```python
from build123d import *

# Parameters (mm, degrees)
EXTRUDE_1_DEPTH        = 20
SKETCH_6_R             = 5
SKETCH_6_R_2           = 2
CUT_EXTRUDE_2_DEPTH    = 2
CHAMFER_2_SIZE         = 4
CHAMFER_3_SIZE         = 0.5
HOLE_WIZARD_M3_1_D     = 2.5
HOLE_WIZARD_M3_1_DEPTH = 7.5
HOLE_WIZARD_M3_1_TIP   = 0.751075774


with BuildPart() as part:
    # 草图1 → 凸台-拉伸1 (new body)
    with BuildSketch(Plane.XY):
        Polygon((0, 3), (0, 0), (-3, 0), (-3, 15), (6, 15), (6, 3), align=None)
    extrude(amount=EXTRUDE_1_DEPTH)

    # 草图6 → 切除-拉伸2 (cut)
    with BuildSketch(Plane.ZY.offset(3)):
        with Locations(Location((10, 9, 0), (0, 0, 270))):
            Circle(SKETCH_6_R)
        with Locations(Location((10, 9, 0), (0, 0, 270))):
            Circle(SKETCH_6_R_2, mode=Mode.SUBTRACT)
    extrude(amount=-CUT_EXTRUDE_2_DEPTH, mode=Mode.SUBTRACT)

    # 倒角2
    chamfer_2_edges = [part.edges().sort_by_distance(p)[0] for p in [
        (1.5, 15, 20),
        (1.5, 15, 0),
    ]]
    chamfer(chamfer_2_edges, length=CHAMFER_2_SIZE)

    # 倒角3
    chamfer_3_edges = [part.edges().sort_by_distance(p)[0] for p in [
        (6, 3, 10),
        (0, 0, 10),
        (-3, 14, 10),
        (-3, 11, 10),
    ]]
    chamfer(chamfer_3_edges, length=CHAMFER_3_SIZE)

    # M3 螺纹孔1
    with Locations(Plane(origin=(0, 3, 0), x_dir=(-1, 0, 0), z_dir=(0, -1, 0))):
        with Locations((-2.5, -5), (-2.5, -15)):
            Hole(HOLE_WIZARD_M3_1_D / 2, depth=HOLE_WIZARD_M3_1_DEPTH)
            with Locations((0, 0, -(HOLE_WIZARD_M3_1_DEPTH + HOLE_WIZARD_M3_1_TIP / 2))):  # 118° drill point
                Cone(0, HOLE_WIZARD_M3_1_D / 2, HOLE_WIZARD_M3_1_TIP, mode=Mode.SUBTRACT)


solid = part.part
```
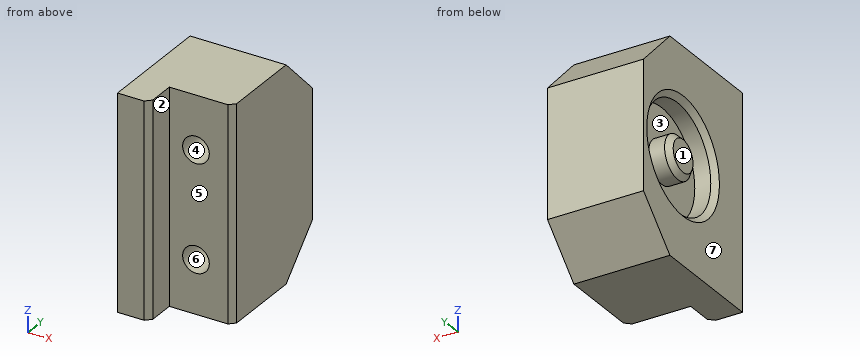
Design review of the part built by this model. Coordinates are the model's own, in mm. Face numbers are marked on the shaded views. A direction names the side the tool comes from. Coordinates: 2 decimals unless noted, no trailing zeros. Loops run counter-clockwise (first coordinate to the right, second up) from the corner with the lowest first, then second, coordinate; pieces in that order, holes last. Notation, with made-up numbers: (-2.5, -31.5) - (8.5, -31.5) arc R20 cw to (8.5, -12.5) - close; hole circle Ø3 at (85, 50.25). An arc over 180 degrees is marked (long way). Use CSV: the item, a comma, the result in double quotes. Start each with the question number.
1) Consider section D-D on y = 3.25. Write out the cut boundary in (x, z), then the cut area to 3 significant figures.
2) Tool access review of the marked faces 1, 2 and 3: name each direction out of +Z, -Z, +X, -X, +Y, -Y from which nothing blocks a thin tool from reaching the whole face with its end or side.
3) Consider section C-C on z = 1.75. Write out the cut boundary in (x, y).
4) Wall thickness on L1, parallel to Z at x = 2.5, y = 6; L2, parallel to X at y = 6.5, z = 15; L3, parallel to Z at x = -1.85, y = 9: over which ranges is each line inside the solid? List them lowest first. Write a range as from..to.
5) Consider section A-A on y = 9. Write out the cut boundary in (x, z), then the cut area to 3 significant figures.
6) Consider section B-B on x = 5. Write out the cut boundary in (y, z).
7) For pin 1 Ø3 at (x, z) = (5, 3) entering from -Y; pin 2 Ø1 at (y, z) = (10.5, 14) entering from -X; pin 3 Ø1.5 at (x, z) = (2.5, 5) entering from -Y, all flat-tipped, find the tip position at first contact; note any pin that passes through.
8) The part is to be moulded in two halves that separate along X. For the marked faces 4, 5, 6 and 7, say which applies: +X half, -X half, draft (parallel to the pull), parting line (faces both ways), or undercut.
Geometry says:
1,outline,"(-3, 0) - (5.75, 0) - (5.75, 20) - (-3, 20) - close; hole circle Ø2.5 at (2.5, 5); hole circle Ø2.5 at (2.5, 15)"
1,area,"165 mm^2"
2,face 1,"+Z, -Z, -X, +Y, -Y"
2,face 2,"+Z, -Z, +X, -Y"
2,face 3,"-X"
3,outline,"(-3, 0) - (-0.5, 0) - (0, 0.5) - (0, 3) - (5.5, 3) - (6, 3.5) - (6, 12.75) - (-3, 12.75) - close"
4,L1,"0..3.75, 6.25..13.75, 16.25..20"
4,L2,"-3..1.25, 3.75..6"
4,L3,"0..5, 8..12, 15..20"
5,outline,"(-3, 0) - (6, 0) - (6, 20) - (-3, 20) - (-3, 15.5) - (-2.5, 15) - (-1, 15) - (-1, 12) - (-2.5, 12) - (-3, 11.5) - (-3, 8.5) - (-2.5, 8) - (-1, 8) - (-1, 5) - (-2.5, 5) - (-3, 4.5) - close; hole circle Ø2.5 at (2.5, 5); hole circle Ø2.5 at (2.5, 15)"
5,area,"158 mm^2"
6,outline,"(3, 0) - (11, 0) - (15, 4) - (15, 16) - (11, 20) - (3, 20) - close"
7,pin 1,"y = 3"
7,pin 2,"x = -1"
7,pin 3,"y = 10.8"
8,face 4,"undercut"
8,face 5,"draft"
8,face 6,"undercut"
8,face 7,"-X half"
